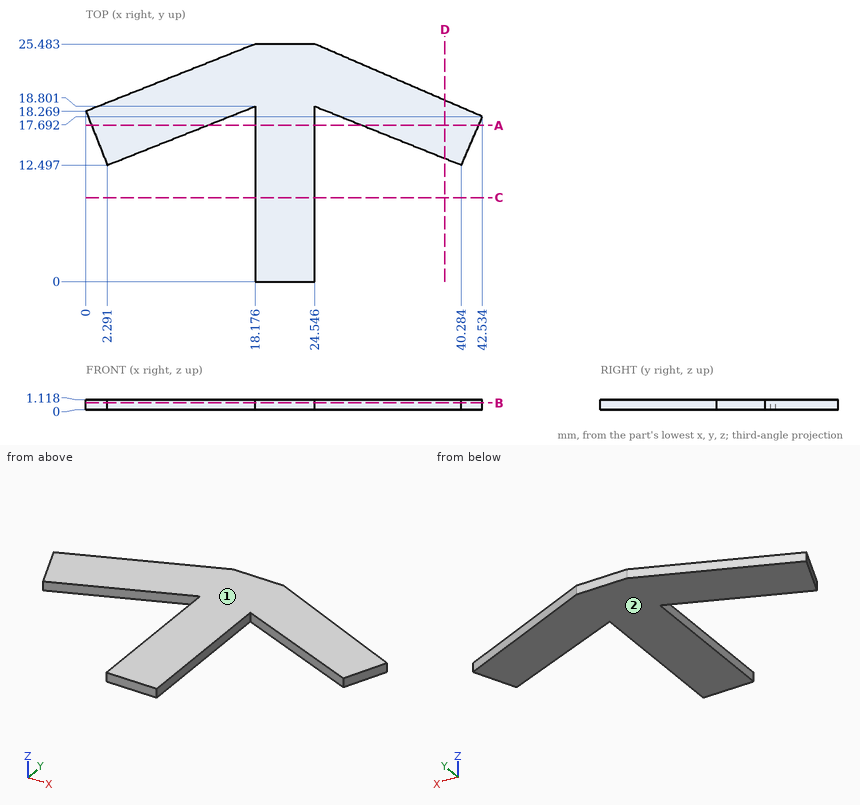
Print and shaded views of the part. All mm, measured from the part's lowest x, y and z. Give positions to 0.01 mm unless a question says otherwise; leave off trailing zeros. Write each loop counter-clockwise with the first axis right and the second up, starting at its lowest first coordinate (ties: lowest second). Pieces come first, ordered by that corner, then holes. Notation, with made-up numbers: (79.25, -16) -> (129.25, -16) arc R12 cw to (129.25, 4) -> close; hole circle Ø4 at (53, 70.25). An arc over 180 degrees is marked (long way). Write item = value, one per line.
(1) Slice it at C-C, the plane y = 9. Give the cut face in (x, z) (1 decimal).
Determined:
outline = (18.2, 0) -> (24.5, 0) -> (24.5, 1.1) -> (18.2, 1.1) -> close
(2) Slice it at B-B, the plane z = 0.75. Give the cut face in (x, y) (1 decimal), then the cut area to 3 significant figures.
Determined:
outline = (0, 18.3) -> (2.3, 12.5) -> (18.2, 18.8) -> (18.2, 0) -> (24.5, 0) -> (24.5, 18.8) -> (40.3, 12.5) -> (42.5, 17.7) -> (24.5, 25.5) -> (18.2, 25.5) -> close
area = 384 mm2
(3) Slice it at D-D, the plane x = 38.5. Give the cut face in (y, z).
Determined:
outline = (13.21, 0) -> (19.44, 0) -> (19.44, 1.12) -> (13.21, 1.12) -> close
(4) Probe line 1 along X through (y, z) = (9, 0.75) (1 decimal); line 2 along Y through (x, z) = (25, 0.1); line 3 along Y through (x, z) = (39, 0.6). List the from-to ranges inside material, lowest first.
Determined:
line_1 = 18.2 to 24.5
line_2 = 18.62 to 25.29
line_3 = 13.01 to 19.22
(5) Mould opens along Z. For the marked faces 1 and 2 say: released by +Z, released by -Z, zero draft, split by the parting line, or undercut.
Determined:
face_1 = released by +Z
face_2 = released by -Z
(6) Slice it at A-A, the plane y = 16.75. Give the cut face in (x, z) (1 decimal).
Determined:
outline = (0.6, 0) -> (13, 0) -> (13, 1.1) -> (0.6, 1.1) -> close; (18.2, 0) -> (24.5, 0) -> (24.5, 1.1) -> (18.2, 1.1) -> close; (29.7, 0) -> (42.1, 0) -> (42.1, 1.1) -> (29.7, 1.1) -> close
